Check sheet for the modelled part. Datum: model origin and axes. Units: mm. A direction names the side the tool comes from. Give positions to 0.01 mm unless a question says otherwise; leave off trailing zeros. Order: outer loops, then holes, each group sorted by start corner. A loop starts at its lowest first (then second) coordinate and runs counter-clockwise, first axis right, second up. Notation, with made-up numbers: (-23.5, 77.5) -> (9.5, 77.5) arc R31 cw to (9.5, 113.5) -> close; hole circle Ø1 at (16, -2.5). An arc over 180 degrees is marked (long way). One line per question, with ' | ' between items.
```python
from build123d import *

# Parameters (mm, degrees)
SKETCH_1_W          = 0.6
SKETCH_1_H          = 10.5
EXTRUDE_1_DEPTH     = 12.5
SKETCH_2_R          = 1.5
SKETCH_3_R          = 1
CUT_EXTRUDE_1_DEPTH = 28.892651362
SKETCH_10_W         = 11.8
SKETCH_10_H         = 6
CUT_EXTRUDE_4_DEPTH = 60


with BuildPart() as part:
    # 草图1 → 拉伸-薄壁1 (new, symmetric)
    with BuildSketch(Plane.XY):
        with Locations((0.3, 5.25)):
            Rectangle(SKETCH_1_W, SKETCH_1_H)
    extrude(amount=EXTRUDE_1_DEPTH, both=True)

    # 扫描1: sweep along a curve in space
    with BuildLine() as sweep_1_path:
        Line((0.6, 10.5, 12.5), (0.6, 10.5, -12.5))
    # 草图2 → 扫描1 (sweep)
    with BuildSketch(Plane.XY.offset(12.5)):
        with Locations((1.5, 10.5)):
            Circle(SKETCH_2_R)
    sweep(path=sweep_1_path.line)

    # 草图3 → 切除-拉伸1 (cut, through all)
    with BuildSketch(Plane.XY.offset(12.5)):
        with Locations((1.5, 10.5)):
            Circle(SKETCH_3_R)
    extrude(amount=-CUT_EXTRUDE_1_DEPTH, mode=Mode.SUBTRACT)

    # 草图10 → 切除-拉伸4 (cut, symmetric)
    with BuildSketch(Plane(origin=(0.6, 0, 0), x_dir=(0, 0, -1), z_dir=(1, 0, 0))):
        with Locations((0, 11)):
            Rectangle(SKETCH_10_W, SKETCH_10_H)
    extrude(amount=CUT_EXTRUDE_4_DEPTH, both=True, mode=Mode.SUBTRACT)

    # 切除-放样1: read off the stored shape, not the designer's step
    # 切除-放样1: loft between two sections, ruled curve by curve
    loft_1_from = [
        Edge.make_bspline([(0, 4.274228258, 10.065269385), (0, 2.143689489, 10.613725902), (0, 1.595232972, 8.483187132), (0, 3.725771742, 7.934730615), (0, 5.856310511, 7.386274098), (0, 6.404767028, 9.516812868), (0, 4.274228258, 10.065269385)], [0, 0, 0, 0, 0.5, 0.5, 0.5, 1, 1, 1, 1], 3, [1, 0.333333333, 0.333333333, 1, 0.333333333, 0.333333333, 1]),
    ]
    loft_1_to = [
        Edge.make_bspline([(0.6, 4.815640724, 10.258860679), (0.6, 2.297919366, 11.890142127), (0.6, 0.666637918, 9.372420769), (0.6, 3.184359276, 7.741139321), (0.6, 5.702080634, 6.109857873), (0.6, 7.333362082, 8.627579231), (0.6, 4.815640724, 10.258860679)], [0, 0, 0, 0, 0.5, 0.5, 0.5, 1, 1, 1, 1], 3, [1, 0.333333333, 0.333333333, 1, 0.333333333, 0.333333333, 1]),
    ]
    loft_1 = Solid(Shell([*[Face.make_surface_from_curves(loft_1_from[k], loft_1_to[k]) for k in range(1)], Face(Wire(loft_1_from)), Face(Wire(loft_1_to))]))
    add(loft_1, mode=Mode.SUBTRACT)

    # 镜向1: 切除-放样1 across plane
    add(loft_1.mirror(Plane.XY), mode=Mode.SUBTRACT)


solid = part.part
```
Q1. Section check D-D (z = 3.75). Enter the section's corners in (x, y), and give its area (3 significant figures).
Result sheet:
outline: (0, 0) -> (0.6, 0) -> (0.6, 8) -> (0, 8) -> close | area: 4.80 mm2
Q2. Access from +Z, -Z, +X, -X, +Y, -Y to the whole of each face (thin tool, end or side, straight path). Record for faces 1 (the face through (0.4, 7.4, 12.5)), 2 (the face through (0.9, 9.5, 5.9)).
Result sheet:
face 1: +Z, +X, -X, +Y, -Y | face 2: +X, -X, +Y
Q3. Section check C-C (z = -9). Count the separate pieces of the cut face and the enclosed holes in it, and give its area (3 significant figures).
Result sheet:
separate pieces: 2 | enclosed holes: 1 | area: 8.18 mm2
Q4. Depth check by flat-ended pin: pin 1 Ø3 at (y, z) = (4.5, -10) entering from +X; pin 2 Ø0.5 at (x, z) = (0.5, -1.5) entering from +Y; pin 3 Ø1.5 at (x, z) = (1, 2.5) entering from -Y. Enter the tip coordinate at first touch or a pass-through.
Result sheet:
pin 1: stops at x = 0.6 | pin 2: stops at y = 8 | pin 3: stops at y = 0
Q5. Section check A-A (x = 1.5). Enter the section's corners in (y, z), and give its area (3 significant figures).
Result sheet:
outline: (9, -12.5) -> (9.5, -12.5) -> (9.5, -5.9) -> (9, -5.9) -> close; (9, 5.9) -> (9.5, 5.9) -> (9.5, 12.5) -> (9, 12.5) -> close; (11.5, -12.5) -> (12, -12.5) -> (12, -5.9) -> (11.5, -5.9) -> close; (11.5, 5.9) -> (12, 5.9) -> (12, 12.5) -> (11.5, 12.5) -> close | area: 13.2 mm2
Q6. Section check B-B (y = 8.25). Enter the section's corners in (x, z), and give its area (3 significant figures).
Result sheet:
outline: (0, -12.5) -> (0.6, -12.5) -> (0.6, -5.9) -> (0, -5.9) -> close; (0, 5.9) -> (0.6, 5.9) -> (0.6, 12.5) -> (0, 12.5) -> close | area: 7.92 mm2
Q7. Thickness scan on line 1 (Z direction, x = 0.5, y = 9.5); line 2 (Y direction, x = 1.5, z = 11.25); line 3 (Y direction, x = 0.45, z = -2.5). Record the ranges inside material, lowest first.
Result sheet:
line 1: z = -12.5 to -5.9, 5.9 to 12.5 | line 2: y = 9 to 9.5, 11.5 to 12 | line 3: y = 0 to 8
Q8. Mould release check, pull along X, two halves, no side actions. Record for faces 3 (the face through (1.37, 11.49, 9.25)), 4 (the face through (0, 5, 0)), 5 (the face through (0.9, 9.5, -5.9)): pulls with the +X half, pulls with the -X half, needs draft (parallel to the pull), parting line crosses it, or undercut.
Result sheet:
face 3: undercut | face 4: pulls with the -X half | face 5: needs draft
